The model under review builds one solid part; all positions refer to its coordinate system, in mm. Face numbers are marked on the shaded views. A direction names the side the tool comes from. Coordinates: 2 decimals unless noted, no trailing zeros. Write each loop counter-clockwise with the first axis right and the second up, starting at its lowest first coordinate (ties: lowest second). Pieces come first, ordered by that corner, then holes. Notation, with made-up numbers: (83, 22) -> (128, 22) arc R24 ccw to (128, 61) -> close; hole circle Ø6 at (-1, -36.5). An arc over 180 degrees is marked (long way). Write each question's results on one line, items separated by ' | '.
```python
from build123d import *

# Parameters (mm, degrees)
BRIDA_BASE1_DEPTH     = 20
CROQUIS5_R            = 1.5
CORTAR_EXTRUIR1_DEPTH = 36.673932989


# Sheet-metal steps are written as plain solids
with BuildPart() as part:
    # Croquis1 → Brida base1 (new body)
    with BuildSketch(Plane.XY):
        with BuildLine():
            Line((-37.721015228, -17.986734349), (-37.721015228, -24.736734349))
            ThreePointArc((-37.721015228, -24.736734349), (-37.42812201, -25.44384113), (-36.721015228, -25.736734349))
            Line((-36.721015228, -25.736734349), (-24.221015228, -25.736734349))
            ThreePointArc((-24.221015228, -25.736734349), (-23.513908447, -25.44384113), (-23.221015228, -24.736734349))
            Line((-23.221015228, -24.736734349), (-23.221015228, -17.986734349))
            Line((-23.221015228, -17.986734349), (-23.721015228, -17.986734349))
            Line((-23.721015228, -17.986734349), (-23.721015228, -24.736734349))
            ThreePointArc((-23.721015228, -24.736734349), (-23.867461838, -25.090287739), (-24.221015228, -25.236734349))
            Line((-24.221015228, -25.236734349), (-36.721015228, -25.236734349))
            ThreePointArc((-36.721015228, -25.236734349), (-37.074568619, -25.090287739), (-37.221015228, -24.736734349))
            Line((-37.221015228, -24.736734349), (-37.221015228, -17.986734349))
            Line((-37.221015228, -17.986734349), (-37.721015228, -17.986734349))
        make_face()
    extrude(amount=BRIDA_BASE1_DEPTH)

    # Croquis5 → Cortar-Extruir1 (cut, through all)
    with BuildSketch(Plane(origin=(-23.221015228, 0, 0), x_dir=(0, 0, -1), z_dir=(1, 0, 0))):
        with Locations((-14, -21.986734349)):
            Circle(CROQUIS5_R)
        with Locations(Location((-6, -21.986734349, 0), (0, 0, 90))):
            Circle(CROQUIS5_R)
    extrude(amount=-CORTAR_EXTRUIR1_DEPTH, mode=Mode.SUBTRACT)


solid = part.part
```
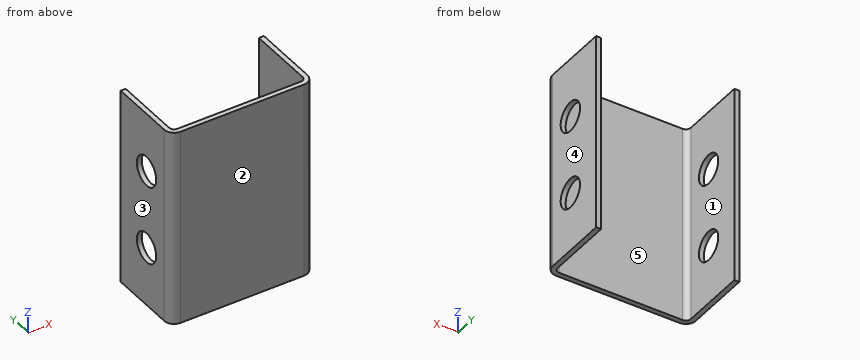
Q1. Clearance check with flat-ended pins moving along their axes: P1, Ø1, axis at x = -36, z = 6, coming from the +Y side; P2, Ø2.5, axis at y = -21.99, z = 6, coming from the -X side. State where each tip first meets the part, or that it passes through.
Solution:
P1: y = -25.24 | P2: through
Q2. Add section B-B (y = -21.75). Write out the cut boundary in (x, z), plus the area to 3 significant figures.
Solution:
outline: (-37.72, 0) -> (-37.22, 0) -> (-37.22, 4.52) -> (-37.72, 4.52) -> close; (-37.72, 7.48) -> (-37.22, 7.48) -> (-37.22, 12.52) -> (-37.72, 12.52) -> close; (-37.72, 15.48) -> (-37.22, 15.48) -> (-37.22, 20) -> (-37.72, 20) -> close; (-23.72, 0) -> (-23.22, 0) -> (-23.22, 4.52) -> (-23.72, 4.52) -> close; (-23.72, 7.48) -> (-23.22, 7.48) -> (-23.22, 12.52) -> (-23.72, 12.52) -> close; (-23.72, 15.48) -> (-23.22, 15.48) -> (-23.22, 20) -> (-23.72, 20) -> close | area: 14.1 mm²
Q3. Add section C-C (y = -19.75). Write out the cut boundary in (x, z).
Solution:
outline: (-37.72, 0) -> (-37.22, 0) -> (-37.22, 20) -> (-37.72, 20) -> close; (-23.72, 0) -> (-23.22, 0) -> (-23.22, 20) -> (-23.72, 20) -> close
Q4. Draft analysis for pull direction X (two halves, no side actions). For the marked faces 1, 2 and 3, state which applies: pulls with the +X half, pulls with the -X half, needs draft (parallel to the pull), parting line crosses it, or undercut.
Solution:
face 1: undercut | face 2: needs draft | face 3: pulls with the -X half
Q5. Add section A-A (z = 14). Write out the cut boundary in (x, y).
Solution:
outline: (-37.72, -24.74) arc R1 ccw to (-36.72, -25.74) -> (-24.22, -25.74) arc R1 ccw to (-23.22, -24.74) -> (-23.22, -23.49) -> (-23.72, -23.49) -> (-23.72, -24.74) arc R0.5 cw to (-24.22, -25.24) -> (-36.72, -25.24) arc R0.5 cw to (-37.22, -24.74) -> (-37.22, -23.49) -> (-37.72, -23.49) -> close; (-37.72, -20.49) -> (-37.22, -20.49) -> (-37.22, -17.99) -> (-37.72, -17.99) -> close; (-23.72, -20.49) -> (-23.22, -20.49) -> (-23.22, -17.99) -> (-23.72, -17.99) -> close
Q6. Machinability: for the marked faces 4 and 5, which of the approach directions +Z, -Z, +X, -X, +Y, -Y give a long, thin tool a straight path to every point of the face, cutting with its end or side? Answer none if there is none.
Solution:
face 4: +Z, -Z, +X, +Y, -Y | face 5: +Z, -Z, +Y
Q7. For line 1 (X direction, y = -22, z = 3); line 2 (Y direction, x = -31, z = 1.75); line 3 (Y direction, x = -23.5, z = 14), list the stretches that pass through material, from the lowest coordinate up. Write a range as from..to.
Solution:
line 1: -37.72..-37.22, -23.72..-23.22 | line 2: -25.74..-25.24 | line 3: -25.43..-23.49, -20.49..-17.99
Q8. Add section D-D (z = 11.25). Write out the cut boundary in (x, y), plus the area to 3 significant figures.
Solution:
outline: (-37.72, -24.74) arc R1 ccw to (-36.72, -25.74) -> (-24.22, -25.74) arc R1 ccw to (-23.22, -24.74) -> (-23.22, -17.99) -> (-23.72, -17.99) -> (-23.72, -24.74) arc R0.5 cw to (-24.22, -25.24) -> (-36.72, -25.24) arc R0.5 cw to (-37.22, -24.74) -> (-37.22, -17.99) -> (-37.72, -17.99) -> close | area: 14.2 mm²
